```python
from build123d import *

# Parameters (mm, degrees)
SKETCH1_R           = 10.287
SKETCH1_R_2         = 6.5405
BOSS_EXTRUDE1_DEPTH = 9.525
SKETCH3_R           = 9.1186
SKETCH3_R_2         = 6.5405
BOSS_EXTRUDE3_DEPTH = 11.0998
SKETCH4_W           = 2.286
SKETCH4_H           = 3.175
CUT_EXTRUDE1_DEPTH  = 14.4399


with BuildPart() as part:
    # Sketch1 → Boss-Extrude1 (new body)
    with BuildSketch(Plane.XY):
        Circle(SKETCH1_R)
        Circle(SKETCH1_R_2, mode=Mode.SUBTRACT)
    extrude(amount=-BOSS_EXTRUDE1_DEPTH)

    # Sketch3 → Boss-Extrude3 (add)
    with BuildSketch(Plane(origin=(0, 0, -9.525), x_dir=(-1, 0, 0), z_dir=(0, 0, -1))):
        Circle(SKETCH3_R)
        with Locations(Location((0, 0, 0), (0, 0, 180))):
            Circle(SKETCH3_R_2, mode=Mode.SUBTRACT)
    extrude(amount=BOSS_EXTRUDE3_DEPTH)

    # Sketch4 → Cut-Extrude1 (cut, symmetric)
    with BuildSketch(Plane(origin=(0, 0, 0), x_dir=(1, 0, 0), z_dir=(0, 1, 0))):
        with Locations((0, 1.5875)):
            Rectangle(SKETCH4_W, SKETCH4_H)
    extrude(amount=CUT_EXTRUDE1_DEPTH, both=True, mode=Mode.SUBTRACT)


solid = part.part
```
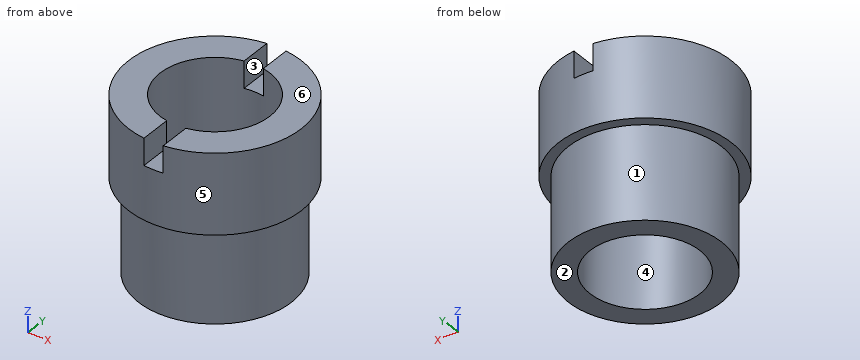
Verification items for the finished model (mm, model axes). Face numbers are marked on the shaded views. A direction names the side the tool comes from. Round coordinates to 2 decimals unless told otherwise and drop trailing zeros. Order: outer loops, then holes, each group sorted by start corner. A loop starts at its lowest first (then second) coordinate and runs counter-clockwise, first axis right, second up. Notation, with made-up numbers: (28, 46) -> (55, 46) arc R28 cw to (55, 76) -> close; hole circle Ø4 at (-8, 62.25). An arc over 180 degrees is marked (long way). Put each result on its own line as item: value. Start each with the question number.
(1) Section check D-D (x = 8.5). Enter the section's corners in (y, z) (3 decimals), then the cut area to 3 significant figures.
(2) Depth check by flat-ended pin: pin 1 Ø6 at (x, y) = (0.5, -4) entering from -Z; pin 2 Ø1.1 at (x, y) = (0, 8.5) entering from +Z (3 decimals); pin 3 Ø8 at (y, z) = (-7, -2.5) entering from -X; pin 4 Ø1 at (y, z) = (9, -1.5) entering from +X. Enter the tip coordinate at first touch or a pass-through.
(3) Section check C-C (z = -10). Enter the section's corners in (x, y), then the cut area to 3 significant figures.
(4) Section check A-A (x = 0). Enter the section's corners in (y, z) (1 decimal), then the cut area to 3 significant figures.
(5) Tool access check on the marked faces 1, 2 and 3. Record the directions out of +Z, -Z, +X, -X, +Y, -Y that give a thin tool (end or side, any length) a straight path to the whole face; none if there is none.
(6) Material ranges on line 1 along Y through (x, z) = (0, -7); line 2 along Y through (x, z) = (0, -13); line 3 along Z through (x, y) = (-8.25, 4.5) (3 decimals), recorded low to high.
(7) Draft check along X on the marked faces 4, 5 and 6. Enter one of: +X half, -X half, draft (parallel to the pull), parting line (faces both ways), or undercut.
(8) Section check B-B (y = 0). Enter the section's corners in (x, z) (1 decimal).
Completed:
1. outline: (-5.794, -9.525) -> (-3.301, -9.525) -> (-3.301, -20.625) -> (3.301, -20.625) -> (3.301, -9.525) -> (5.794, -9.525) -> (5.794, 0) -> (-5.794, 0) -> close
1. area: 184 mm2
2. pin 1: stops at z = -20.62
2. pin 2: stops at z = -3.175
2. pin 3: stops at x = -9.84
2. pin 4: stops at x = 5.79
3. outline: circle Ø18.24 at (0, 0); hole circle Ø13.08 at (0, 0)
3. area: 127 mm2
4. outline: (-10.3, -9.5) -> (-9.1, -9.5) -> (-9.1, -20.6) -> (-6.5, -20.6) -> (-6.5, -3.2) -> (-10.3, -3.2) -> close; (6.5, -20.6) -> (9.1, -20.6) -> (9.1, -9.5) -> (10.3, -9.5) -> (10.3, -3.2) -> (6.5, -3.2) -> close
4. area: 105 mm2
5. face 1: -Z
5. face 2: -Z, +X, -X, +Y, -Y
5. face 3: +Z, +Y, -Y
6. line 1: y = -10.29 to -6.54, 6.54 to 10.29
6. line 2: y = -9.12 to -6.54, 6.54 to 9.12
6. line 3: z = -9.525 to 0
7. face 4: undercut
7. face 5: parting line
7. face 6: draft
8. outline: (-10.3, -9.5) -> (-9.1, -9.5) -> (-9.1, -20.6) -> (-6.5, -20.6) -> (-6.5, 0) -> (-10.3, 0) -> close; (6.5, -20.6) -> (9.1, -20.6) -> (9.1, -9.5) -> (10.3, -9.5) -> (10.3, 0) -> (6.5, 0) -> close
